from build123d import *

# Parameters (mm, degrees)
F0_W          = 152.4
F0_H          = 101.6
F1_DEPTH      = 5.08
F2_W          = 7.62
F2_H          = 101.6
F3_DEPTH      = 10.16
F4_T1_DEPTH   = 127
F5_W          = 7.62
F5_H          = 101.6
F6_DEPTH      = 7.62
F7_T1_DEPTH   = 127
F8_W          = 8.89
F8_H          = 101.6
F9_DEPTH      = 10.16
F10_T1_DEPTH  = 127
F11_W         = 101.6
F11_H         = 43.9456890713
F12_DEPTH     = 25.4
F13_T1_DEPTH  = 5.08
F13_T3_DEPTH  = 30.48
F13_T5_DEPTH  = 35.56
F13_T7_DEPTH  = 33.02
F14_T1_DEPTH  = 36.2882991577
F14_T3_DEPTH  = 33.7482991577
F14_T5_DEPTH  = 64.1381350342
F14_T7_DEPTH  = 64.1318649658
F14_T12_DEPTH = 90.2664341919
F14_T17_DEPTH = 90.2601641236
F15_W         = 11.43
F15_H         = 11.43
F16_DEPTH     = 6.35
F17_W         = 11.43
F17_H         = 11.43
F18_DEPTH     = 6.35
F19_W         = 11.43
F19_H         = 3.175
F20_DEPTH     = 5.08
F21_W         = 11.43
F21_H         = 3.175
F22_DEPTH     = 5.08
F23_W         = 101.4830252707
F23_H         = 42.7652306713
F24_DEPTH     = 25.4


# Not quite as in the source:
# - a fillet or chamfer that OpenCascade refuses, or shapes differently, is made with other operations: its cross-section is extruded or revolved along the edge and cut away or added


with BuildPart() as f1:
    # F0 (on Top) → F1 (new body)
    with BuildSketch(Plane.XY):
        Rectangle(F0_W, F0_H)
    extrude(amount=F1_DEPTH)

    # F2 (on face) → F3 (join)
    with BuildSketch(Plane(origin=(0, 0, 0), x_dir=(1, 0, 0), z_dir=(0, 0, -1))):
        with Locations((-72.39, 0)):
            Rectangle(F2_W, F2_H)
    extrude(amount=F3_DEPTH)

    # F4: fillet of radius 5.08 on 2 edges, made by hand

    # F4_s2 → F4_t1 (cut)
    with BuildSketch(Plane.XZ.offset(-63.5)):
        with BuildLine():
            ThreePointArc((-71.12, -10.16), (-74.7121024484, -8.6721024484), (-76.2, -5.08))
            Line((-76.2, -5.08), (-76.2, -10.16))
            Line((-76.2, -10.16), (-71.12, -10.16))
        make_face()
        with BuildLine():
            ThreePointArc((-68.58, -5.08), (-70.0678975516, -8.6721024484), (-73.66, -10.16))
            Line((-73.66, -10.16), (-68.58, -10.16))
            Line((-68.58, -10.16), (-68.58, -5.08))
        make_face()
    extrude(amount=F4_T1_DEPTH, mode=Mode.SUBTRACT)

    # F5 (on face) → F6 (join)
    with BuildSketch(Plane(origin=(0, 0, 0), x_dir=(1, 0, 0), z_dir=(0, 0, -1))):
        with Locations((72.39, 0)):
            Rectangle(F5_W, F5_H)
    extrude(amount=F6_DEPTH)

    # F7: fillet of radius 5.08 on 2 edges, made by hand

    # F7_s2 → F7_t1 (cut)
    with BuildSketch(Plane.XZ.offset(-63.5)):
        with BuildLine():
            ThreePointArc((76.2, -2.54), (74.7121024484, -6.1321024484), (71.12, -7.62))
            Line((71.12, -7.62), (76.2, -7.62))
            Line((76.2, -7.62), (76.2, -2.54))
        make_face()
        with BuildLine():
            ThreePointArc((73.66, -7.62), (70.0678975516, -6.1321024484), (68.58, -2.54))
            Line((68.58, -2.54), (68.58, -7.62))
            Line((68.58, -7.62), (73.66, -7.62))
        make_face()
    extrude(amount=F7_T1_DEPTH, mode=Mode.SUBTRACT)

    # F8 (on face) → F9 (join)
    with BuildSketch(Plane(origin=(0, 0, 0), x_dir=(1, 0, 0), z_dir=(0, 0, -1))):
        with Locations((-0.0031350342, 0)):
            Rectangle(F8_W, F8_H)
    extrude(amount=F9_DEPTH)

    # F10: fillet of radius 5.08 on 2 edges, made by hand

    # F10_s2 → F10_t1 (cut)
    with BuildSketch(Plane.XZ.offset(-63.5)):
        with BuildLine():
            ThreePointArc((-4.4481350342, -5.08), (-2.9602374826, -8.6721024484), (0.6318649658, -10.16))
            Line((0.6318649658, -10.16), (-4.4481350342, -10.16))
            Line((-4.4481350342, -10.16), (-4.4481350342, -5.08))
        make_face()
        with BuildLine():
            ThreePointArc((4.4418649658, -5.08), (2.9539674142, -8.6721024484), (-0.6381350342, -10.16))
            Line((-0.6381350342, -10.16), (4.4418649658, -10.16))
            Line((4.4418649658, -10.16), (4.4418649658, -5.08))
        make_face()
    extrude(amount=F10_T1_DEPTH, mode=Mode.SUBTRACT)

    # F11 (on face) → F12 (cut)
    with BuildSketch(Plane.XY.offset(5.08)):
        with Locations((0, 28.8271554643)):
            Rectangle(F11_W, F11_H)
    extrude(amount=-F12_DEPTH, mode=Mode.SUBTRACT)

    # F13: fillet of radius 5.08 on 5 edges, made by hand

    # F13_s2 → F13_t1 (join)
    with BuildSketch(Plane.XY):
        with BuildLine():
            ThreePointArc((50.8, 11.9343109287), (49.3121024484, 8.3422084803), (45.72, 6.8543109287))
            Line((45.72, 6.8543109287), (50.8, 6.8543109287))
            Line((50.8, 6.8543109287), (50.8, 11.9343109287))
        make_face()
    extrude(amount=F13_T1_DEPTH)

    # F13_s4 → F13_t3 (cut)
    with BuildSketch(Plane.XY.offset(-12.7)):
        with BuildLine():
            ThreePointArc((-55.88, 50.8), (-52.2878975516, 49.3121024484), (-50.8, 45.72))
            Line((-50.8, 45.72), (-50.8, 50.8))
            Line((-50.8, 50.8), (-55.88, 50.8))
        make_face()
        with BuildLine():
            ThreePointArc((55.88, 50.8), (52.2878975516, 49.3121024484), (50.8, 45.72))
            Line((50.8, 45.72), (50.8, 50.8))
            Line((50.8, 50.8), (55.88, 50.8))
        make_face()
    extrude(amount=F13_T3_DEPTH, mode=Mode.SUBTRACT)

    # F13_s6 → F13_t5 (cut)
    with BuildSketch(Plane.XY.offset(-17.78)):
        with BuildLine():
            ThreePointArc((-76.2, 45.72), (-74.7121024484, 49.3121024484), (-71.12, 50.8))
            Line((-71.12, 50.8), (-76.2, 50.8))
            Line((-76.2, 50.8), (-76.2, 45.72))
        make_face()
    extrude(amount=F13_T5_DEPTH, mode=Mode.SUBTRACT)

    # F13_s8 → F13_t7 (cut)
    with BuildSketch(Plane.XY.offset(-15.24)):
        with BuildLine():
            ThreePointArc((71.12, 50.8), (74.7121024484, 49.3121024484), (76.2, 45.72))
            Line((76.2, 45.72), (76.2, 50.8))
            Line((76.2, 50.8), (71.12, 50.8))
        make_face()
    extrude(amount=F13_T7_DEPTH, mode=Mode.SUBTRACT)

    # F14: chamfer of 5.08 on 4 edges, made by hand

    # F14_s2 → F14_t1 (cut)
    with BuildSketch(Plane.XY.offset(-18.1441495789)):
        Polygon((-71.12, -50.8), (-76.2, -45.72), (-76.2, -50.8), align=None)
    extrude(amount=F14_T1_DEPTH, mode=Mode.SUBTRACT)

    # F14_s4 → F14_t3 (cut)
    with BuildSketch(Plane.XY.offset(-15.6041495789)):
        Polygon((71.12, -50.8), (76.2, -45.72), (76.2, -50.8), align=None)
    extrude(amount=F14_T3_DEPTH, mode=Mode.SUBTRACT)

    # F14_s6 → F14_t5 (cut)
    with BuildSketch(Plane.YZ.offset(4.4418649658)):
        Polygon((-45.72, 0), (-50.8, 5.08), (-50.8, 0), align=None)
    extrude(amount=F14_T5_DEPTH, mode=Mode.SUBTRACT)

    # F14_s8 → F14_t7 (cut)
    with BuildSketch(Plane.YZ.offset(-68.58)):
        Polygon((-50.8, 5.08), (-45.72, 0), (-50.8, 0), align=None)
    extrude(amount=F14_T7_DEPTH, mode=Mode.SUBTRACT)


with BuildPart() as f14_tool10:
    # F14_s11 → F14_t12 (new body)
    with BuildSketch(Plane.YZ.offset(-8.622284613)):
        Polygon((-45.72, 0), (-50.8, 5.08), (-50.8, 0), align=None)
    extrude(amount=F14_T12_DEPTH)

    split(bisect_by=Plane.YZ.offset(-4.4481350342), keep=Keep.BOTTOM)


with BuildPart() as f1_1:
    add(f1.part)

    # F14_t9: cut F14_tool10
    add(f14_tool10.part, mode=Mode.SUBTRACT)


with BuildPart() as f14_tool15:
    # F14_s16 → F14_t17 (new body)
    with BuildSketch(Plane.YZ.offset(-81.6441495789)):
        Polygon((-50.8, 5.08), (-45.72, 0), (-50.8, 0), align=None)
    extrude(amount=F14_T17_DEPTH)

    split(bisect_by=Plane.YZ.offset(4.4418649658), keep=Keep.TOP)


with BuildPart() as f1_2:
    add(f1_1.part)

    # F14_t14: cut F14_tool15
    add(f14_tool15.part, mode=Mode.SUBTRACT)

    # F15 (on face) → F16 (join)
    with BuildSketch(Plane.XY.offset(5.08)):
        with Locations((63.0153976381, 16.3576488795)):
            Rectangle(F15_W, F15_H)
    extrude(amount=F16_DEPTH)

    # F17 (on face) → F18 (join)
    with BuildSketch(Plane.XY.offset(5.08)):
        with Locations((-63.7673679739, 17.1340169625)):
            Rectangle(F17_W, F17_H)
    extrude(amount=F18_DEPTH)

    # F19 (on face) → F20 (join)
    with BuildSketch(Plane(origin=(-69.4823679739, 0, 0), x_dir=(0, -1, 0), z_dir=(-1, 0, 0))):
        with Locations((-17.1340169625, 9.8425)):
            Rectangle(F19_W, F19_H)
    extrude(amount=F20_DEPTH)

    # F21 (on face) → F22 (join)
    with BuildSketch(Plane.YZ.offset(68.7303976381)):
        with Locations((16.3576488795, 9.8425)):
            Rectangle(F21_W, F21_H)
    extrude(amount=F22_DEPTH)

    # F23 (on face) → F24 (cut)
    with BuildSketch(Plane.XY.offset(5.08)):
        with Locations((-0.0584873646, -9.448304407)):
            Rectangle(F23_W, F23_H)
    extrude(amount=-F24_DEPTH, mode=Mode.SUBTRACT)


solid = f1_2.part
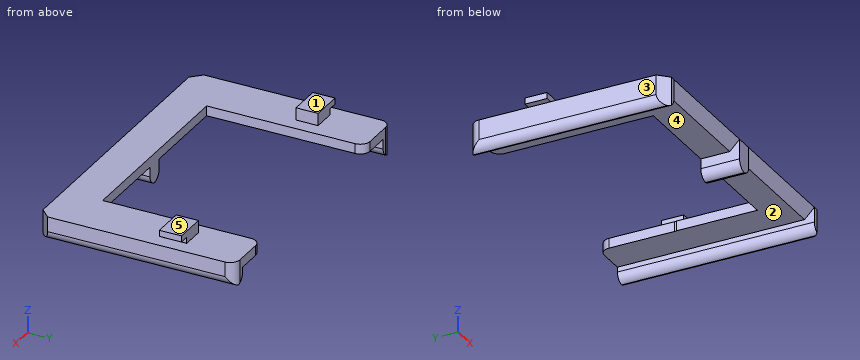
Read the model definition and answer for the solid it produces. Units are mm, in the model's axes. Face numbers are marked on the shaded views. A direction names the side the tool comes from. Round coordinates to 2 decimals unless told otherwise and drop trailing zeros. Write each loop counter-clockwise with the first axis right and the second up, starting at its lowest first coordinate (ties: lowest second). Pieces come first, ordered by that corner, then holes.
1. The part is cut by section C-C, the plane z = 2.75. Determine the outline of the cut face in (x, y).
2. Straight lines are drawn through the part: L1, parallel to X at y = -15.5, z = -2.25; L2, parallel to X at y = -18.5, z = 4.5; L3, parallel to Z at x = -64, y = 44. For each, find the intervals that lie inside material, in ascending order.
3. Which of the six approach directions +Z, -Z, +X, -X, +Y, -Y give full straight-line access (tool end or side, diameter ignored) to the marked faces 4 and 5?
4. The part is cut by section B-B, the plane x = 67. Determine the outline of the cut face in (y, z).
5. The part is cut by section A-A, the plane y = -4. Determine the outline of the cut face in (x, z).
6. The part is cut by section D-D, the plane y = 25. Determine the outline of the cut face in (x, z).
7. Given pin 1 Ø1.6 at (y, z) = (15, 10.5) entering from -X; pin 2 Ø3 at (x, z) = (-19.5, 1) entering from +Y; pin 3 Ø2.5 at (y, z) = (14, 10.5) entering from +X, each flat-ended and moving along its own axis, determine where each tip first touches the part or whether it passes through.
8. Determine the mould class of the marked faces 1, 2 and 3 for opening direction X: pulls with the +X half, pulls with the -X half, needs draft (parallel to the pull), parting line crosses it, or undercut.
Values:
1. outline: (-76.2, -45.72) - (-71.12, -50.8) - (-68.58, -50.8) - (-68.58, -48.47) - (-4.45, -48.47) - (-4.45, -50.8) - (4.44, -50.8) - (4.44, -48.47) - (68.58, -48.47) - (68.58, -50.8) - (71.12, -50.8) - (76.2, -45.72) - (76.2, 45.72) arc R5.08 ccw to (71.12, 50.8) - (55.88, 50.8) arc R5.08 ccw to (50.8, 45.72) - (50.8, 11.93) arc R5.08 cw to (50.68, 10.85) - (50.68, -30.83) - (-50.8, -30.83) - (-50.8, 45.72) arc R5.08 ccw to (-55.88, 50.8) - (-71.12, 50.8) arc R5.08 ccw to (-76.2, 45.72) - close
2. L1: x = -76.2 to -68.58, 68.58 to 76.2
2. L2: x = -76.2 to -50.8, 50.68 to 76.2
2. L3: z = 0 to 5.08
3. face 4: -Z, +Y, -Y
3. face 5: +Z, +X, -X, +Y, -Y
4. outline: (-50.8, 5.08) - (-45.72, 0) - (50.8, 0) - (50.8, 5.08) - (22.07, 5.08) - (22.07, 11.43) - (10.64, 11.43) - (10.64, 5.08) - close
5. outline: (-76.2, -5.08) arc R5.08 ccw to (-72.39, -10) arc R5.08 ccw to (-68.58, -5.08) - (-68.58, 0) - (-50.8, 0) - (-50.8, 5.08) - (-76.2, 5.08) - close; (50.68, 0) - (68.58, 0) - (68.58, -2.54) arc R5.08 ccw to (72.39, -7.46) arc R5.08 ccw to (76.2, -2.54) - (76.2, 5.08) - (50.68, 5.08) - close
6. outline: (-76.2, -5.08) arc R5.08 ccw to (-72.39, -10) arc R5.08 ccw to (-68.58, -5.08) - (-68.58, 0) - (-50.8, 0) - (-50.8, 5.08) - (-76.2, 5.08) - close; (50.8, 0) - (68.58, 0) - (68.58, -2.54) arc R5.08 ccw to (72.39, -7.46) arc R5.08 ccw to (76.2, -2.54) - (76.2, 5.08) - (50.8, 5.08) - close
7. pin 1: stops at x = -74.56
7. pin 2: stops at y = -30.83
7. pin 3: stops at x = 73.81
8. face 1: needs draft
8. face 2: undercut
8. face 3: pulls with the -X half
